```python
from build123d import *

# Parameters (mm, degrees)
SKETCH1_W           = 150
SKETCH1_H           = 150
BOSS_EXTRUDE1_DEPTH = 10
SKETCH3_W           = 100
SKETCH3_H           = 50
BOSS_EXTRUDE2_DEPTH = 50
CUT_EXTRUDE1_DEPTH  = 205.266982158
SKETCH5_W           = 100
SKETCH5_H           = 50
CUT_EXTRUDE2_DEPTH  = 218.944947177
SKETCH7_W           = 120
SKETCH7_H           = 70
BOSS_EXTRUDE6_DEPTH = 50
BOSS_EXTRUDE7_DEPTH = 100
SKETCH9_W           = 100
SKETCH9_H           = 40
CUT_EXTRUDE4_DEPTH  = 40
BOSS_EXTRUDE8_DEPTH = 100
CUT_EXTRUDE5_DEPTH  = 211.535032714
SHELL1_START        = 35
SHELL1_DEPTH        = 80
SKETCH12_R          = 2.5
CUT_EXTRUDE6_DEPTH  = 221.45407685


# Read off the part's stored shape, not the designer's step: Shell1
with BuildPart() as part:
    # Sketch1 → Boss-Extrude1 (new body)
    with BuildSketch(Plane(origin=(0, 0, 0), x_dir=(1, 0, 0), z_dir=(0, 1, 0))):
        with Locations((75, 75)):
            Rectangle(SKETCH1_W, SKETCH1_H)
    extrude(amount=BOSS_EXTRUDE1_DEPTH)

    # Sketch3 → Boss-Extrude2 (add)
    with BuildSketch(Plane(origin=(0, 10, 0), x_dir=(1, 0, 0), z_dir=(0, 1, 0))):
        with Locations((75, 100)):
            Rectangle(SKETCH3_W, SKETCH3_H)
    extrude(amount=BOSS_EXTRUDE2_DEPTH)

    # Sketch4 → Cut-Extrude1 (cut, through all)
    with BuildSketch(Plane.ZY.offset(-25)):
        Polygon((-125, 60), (-75, 10), (-75, 60), align=None)
    extrude(amount=-CUT_EXTRUDE1_DEPTH, mode=Mode.SUBTRACT)

    # Sketch5 → Cut-Extrude2 (cut, through all)
    with BuildSketch(Plane(origin=(0, 10, 0), x_dir=(1, 0, 0), z_dir=(0, 1, 0))):
        with Locations((75, 50)):
            Rectangle(SKETCH5_W, SKETCH5_H)
    extrude(amount=-CUT_EXTRUDE2_DEPTH, mode=Mode.SUBTRACT)

    # Sketch7 → Boss-Extrude6 (add)
    with BuildSketch(Plane.XZ):
        with Locations((75, -50)):
            Rectangle(SKETCH7_W, SKETCH7_H)
    extrude(amount=BOSS_EXTRUDE6_DEPTH)

    # Sketch6 → Boss-Extrude7 (add)
    with BuildSketch(Plane(origin=(25, 0, 0), x_dir=(0, 0, -1), z_dir=(1, 0, 0))):
        Polygon((75, 0), (75, 10), (65, 0), align=None)
    extrude(amount=BOSS_EXTRUDE7_DEPTH)

    # Sketch9 → Cut-Extrude4 (cut)
    with BuildSketch(Plane(origin=(0, 0, 0), x_dir=(1, 0, 0), z_dir=(0, 1, 0))):
        with Locations((75, 45)):
            Rectangle(SKETCH9_W, SKETCH9_H)
    extrude(amount=-CUT_EXTRUDE4_DEPTH, mode=Mode.SUBTRACT)

    # Sketch10 → Boss-Extrude8 (add)
    with BuildSketch(Plane(origin=(25, 0, 0), x_dir=(0, 0, -1), z_dir=(1, 0, 0))):
        Polygon((65, 0), (25, -40), (65, -40), align=None)
    extrude(amount=BOSS_EXTRUDE8_DEPTH)

    # Sketch11 → Cut-Extrude5 (cut, through all)
    with BuildSketch(Plane(origin=(135, 0, 0), x_dir=(0, 0, -1), z_dir=(1, 0, 0))):
        Polygon((85, 0), (85, -50), (35, -50), align=None)
    extrude(amount=-CUT_EXTRUDE5_DEPTH, mode=Mode.SUBTRACT)

    # Shell1 outline → Shell1 (cut)
    with BuildSketch(Plane.YZ.offset(SHELL1_START)):
        Polygon((45.857864376, -125), (10, -89.142135624), (10, -125), align=None)
    extrude(amount=SHELL1_DEPTH, mode=Mode.SUBTRACT)

    # Sketch12 → Cut-Extrude6 (cut, through all)
    with BuildSketch(Plane.XZ):
        with Locations(Location((125, -140, 0), (0, 0, 270))):
            Circle(SKETCH12_R)
        with Locations(Location((75, -140, 0), (0, 0, 270))):
            Circle(SKETCH12_R)
        with Locations(Location((25, -140, 0), (0, 0, 270))):
            Circle(SKETCH12_R)
        with Locations(Location((125, -5, 0), (0, 0, 270))):
            Circle(SKETCH12_R)
        with Locations(Location((75, -5, 0), (0, 0, 270))):
            Circle(SKETCH12_R)
        with Locations(Location((25, -5, 0), (0, 0, 270))):
            Circle(SKETCH12_R)
    extrude(amount=-CUT_EXTRUDE6_DEPTH, mode=Mode.SUBTRACT)


solid = part.part
```
The listing builds one solid part. Answer for the finished solid, in the listing's coordinates (mm). A direction names the side the tool comes from. Coordinates: 2 decimals unless noted, no trailing zeros. Loops run counter-clockwise (first coordinate to the right, second up) from the corner with the lowest first, then second, coordinate; pieces in that order, holes last. Notation, with made-up numbers: M -36,48 L -14,48 A19 ccw -14,76 Z; hole C 0,79.5 d11. An arc over 180 degrees is marked long. Answer as a JSON object with one key per item and string values. Group by question number.
Item 1: Section D-D (z = -117.5) is taken. Write down the section's boundary in (x, y), and give its area (3 significant figures).
Item 2: Section A-A (z = -140) is taken. Write down the section's boundary in (x, y).
Item 3: Section B-B (x = 75) is taken. Write down the section's boundary in (y, z).
Item 4: Section C-C (y = -32) is taken. Write down the section's boundary in (x, z).
Item 5: Consider L1, parallel to X at y = 7, z = -140; L2, parallel to Z at x = 74, y = 3; L3, parallel to Y at x = 50, z = -129. Determine where each line is inside the solid, lowest interval first.
Item 6: Which of the six approach directions +Z, -Z, +X, -X, +Y, -Y give full straight-line access (tool end or side, diameter ignored) to faces 1 (the face through (35, 20, -115)), 2 (the face through (125, -9, -44)), 3 (the face through (74, -25, -15)), 4 (the face through (76, -25, -60)), 5 (the face through (125, 24, -111))?
Item 7: Determine the mould class of faces 6 (the face through (74, 5, 0)), 7 (the face through (15, -19, -43)), 8 (the face through (125.751, 4.93, -142.385)) for opening direction X: +X half, -X half, draft (parallel to the pull), parting line (faces both ways), or undercut.
Item 8: Each of these flat-tipped pins is pushed along its axis until it touches: P1, Ø4, axis at x = 132.5, z = -25.5, coming from the +Y side; P2, Ø6, axis at x = 39, y = 35.5, coming from the +Z side; P3, Ø4, axis at x = 130, y = -22.5, coming from the -Z side; P4, Ø4, axis at x = 125, z = -140, coming from the -Y side. Where does it stop, or does it pass through?
Solved:
{
 "1": {"outline": "M 0,0 L 150,0 L 150,10 L 125,10 L 125,52.5 L 25,52.5 L 25,10 L 0,10 Z; hole M 35,10 L 115,10 L 115,38.36 L 35,38.36 Z", "area": "3,480 mm2"},
 "2": {"outline": "M 0,0 L 22.5,0 L 22.5,10 L 0,10 Z; M 27.5,0 L 72.5,0 L 72.5,10 L 27.5,10 Z; M 77.5,0 L 122.5,0 L 122.5,10 L 77.5,10 Z; M 127.5,0 L 150,0 L 150,10 L 127.5,10 Z"},
 "3": {"outline": "M -50,-35 L 0,-85 L 0,-137.5 L 10,-137.5 L 10,-89.14 L 45.86,-125 L 60,-125 L -40,-25 L 10,-25 L 10,-7.5 L 0,-7.5 L 0,-15 L -50,-15 Z; M 0,-150 L 10,-150 L 10,-142.5 L 0,-142.5 Z; M 0,-2.5 L 10,-2.5 L 10,0 L 0,0 Z"},
 "4": {"outline": "M 15,-53 L 135,-53 L 135,-15 L 15,-15 Z; hole M 25,-33 L 125,-33 L 125,-25 L 25,-25 Z"},
 "5": {"L1": "x = 0 to 22.5, 27.5 to 72.5, 77.5 to 122.5, 127.5 to 150", "L2": "z = -150 to -142.29, -137.71 to -68, -25 to -7.29, -2.71 to 0", "L3": "y = 0 to 10"},
 "6": {"face 1": "-Z", "face 2": "+Y", "face 3": "+Z, +X, -X, -Y", "face 4": "-Z, +X, -X, -Y", "face 5": "+Z, -Z, +X, +Y"},
 "7": {"face 6": "draft", "face 7": "-X half", "face 8": "undercut"},
 "8": {"P1": "stops at y = 10", "P2": "stops at z = -97.5", "P3": "stops at z = -64.5", "P4": "passes through"}
}
